Design review of the part built by this model. Coordinates are the model's own, in mm. Give positions to 0.01 mm unless a question says otherwise; leave off trailing zeros. Order: outer loops, then holes, each group sorted by start corner. A loop starts at its lowest first (then second) coordinate and runs counter-clockwise, first axis right, second up.
```python
from build123d import *

# Parameters (mm, degrees)
F0_W     = 1.5875
F0_H     = 55.5625
F1_DEPTH = 33.3375
F0_W_2   = 31.75
F2_DEPTH = 1.5875


with BuildPart() as f1:
    # F0 (on Top) → F1 (new body)
    with BuildSketch(Plane.XY):
        Polygon((1.5875, 0), (0, 0), (-31.75, 0), (-33.3375, 0), (-33.3375, -1.5875), (101.6, -1.5875), (101.6, 0), (100.0125, 0), (68.2625, 0), (66.675, 0), (34.925, 0), (33.3375, 0), align=None)
        with Locations((-32.54375, 27.78125)):
            Rectangle(F0_W, F0_H)
        Polygon((-31.75, 55.5625), (0, 55.5625), (1.5875, 55.5625), (33.3375, 55.5625), (34.925, 55.5625), (66.675, 55.5625), (68.2625, 55.5625), (100.0125, 55.5625), (101.6, 55.5625), (101.6, 57.15), (-33.3375, 57.15), (-33.3375, 55.5625), align=None)
        with Locations((100.80625, 27.78125)):
            Rectangle(F0_W, F0_H)
        with Locations((0.79375, 27.78125)):
            Rectangle(F0_W, F0_H)
        with Locations((34.13125, 27.78125)):
            Rectangle(F0_W, F0_H)
        with Locations((67.46875, 27.78125)):
            Rectangle(F0_W, F0_H)
    extrude(amount=F1_DEPTH)

    # F0 (on Top) → F2 (join)
    with BuildSketch(Plane.XY):
        with Locations((-15.875, 27.78125)):
            Rectangle(F0_W_2, F0_H)
        with Locations((17.4625, 27.78125)):
            Rectangle(F0_W_2, F0_H)
        with Locations((84.1375, 27.78125)):
            Rectangle(F0_W_2, F0_H)
        with Locations((50.8, 27.78125)):
            Rectangle(F0_W_2, F0_H)
    extrude(amount=F2_DEPTH)


solid = f1.part
```
1. Draft analysis for pull direction X (two halves, no side actions). For faces 1 (the face through (35, 57.15, 16)), 2 (the face through (101.6, 27, 16)), 3 (the face through (84, 55.562, 17)), state which applies: pulls with the +X half, pulls with the -X half, needs draft (parallel to the pull), parting line crosses it, or undercut.
Recorded:
face 1: needs draft
face 2: pulls with the +X half
face 3: undercut
2. For pin 1 (9.5 mm diameter, centred on x = 19, y = 32, fed in from +Z), flat-tipped, find the tip position at first contact; note if it passes through.
Recorded:
pin 1: stops at z = 1.59
3. Take a section at B-B (x = 81.5). State the section outline as (y, z) points.
Recorded:
outline: (-1.59, 0) - (57.15, 0) - (57.15, 33.34) - (55.56, 33.34) - (55.56, 1.59) - (0, 1.59) - (0, 33.34) - (-1.59, 33.34) - close
4. Take a section at A-A (z = 24). State how many separate pieces and enclosed holes the cut face has, then the cut area to 3 significant figures.
Recorded:
separate pieces: 1
enclosed holes: 4
area: 869 mm2
5. For line 1 along Y through (x, z) = (-11, 28); line 2 along Z through (x, y) = (32, 25), list the stretches that pass through material, from the lowest coordinate up.
Recorded:
line 1: y = -1.59 to 0, 55.56 to 57.15
line 2: z = 0 to 1.59
